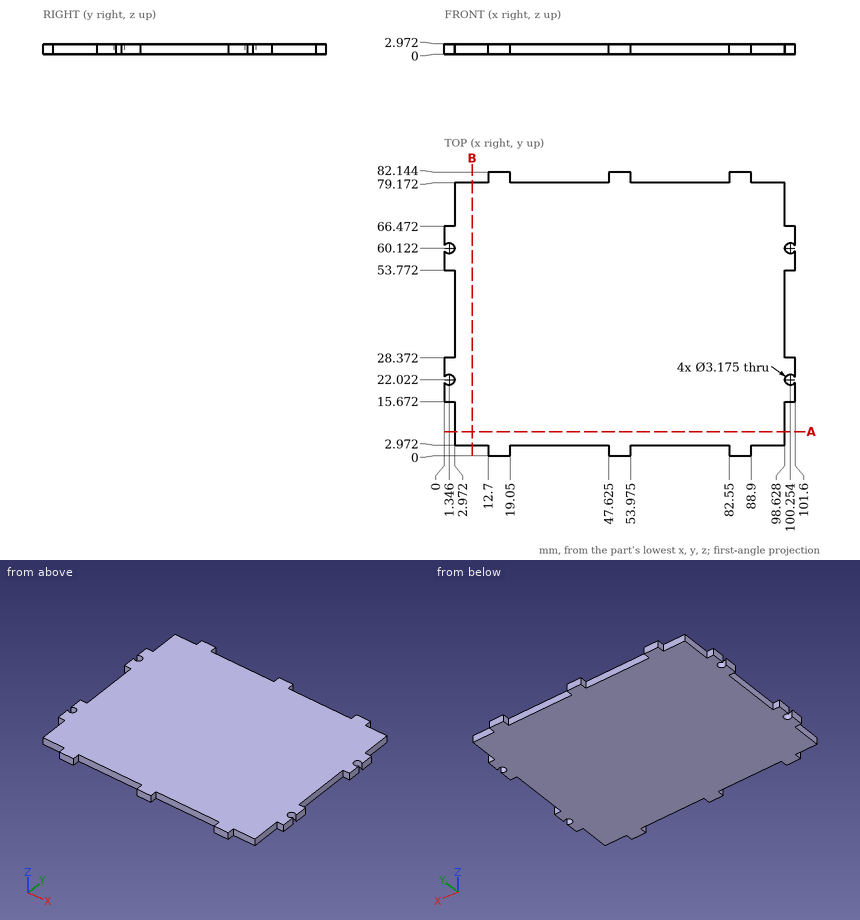
Print and shaded views of the part. All mm, measured from the part's lowest x, y and z. Coordinates: 2 decimals unless noted, no trailing zeros. Write each loop counter-clockwise with the first axis right and the second up, starting at its lowest first coordinate (ties: lowest second). Pieces come first, ordered by that corner, then holes.
(1) Cut at A-A, the plane y = 7. List the corners of the cut face in (x, z).
(2) Drill centre lines: probe 1 along X at (y, z) = (69, 1.9); probe 2 along Y at (x, z) = (60.5, 1.1). Where is each one in solid material? Low to high.
(3) Flat gauge pins, fed straight in: pin 1 (1.5 mm diameter, centred on y = 1.5, z = 2, fed in from -X); pin 2 (1.5 mm diameter, centred on x = 100, z = 1, fed in from -Y); pin 3 (2 mm diameter, centred on x = 80.5, y = 28.5, fed in from -Z); pin 4 (1.5 mm diameter, centred on y = 36.5, z = 2, fed in from -X). Where does each tip first touch, or does it go through?
(4) Cut at B-B, the plane x = 8. List the corners of the cut face in (y, z).
Geometry says:
1. outline: (2.97, 0) - (98.63, 0) - (98.63, 2.97) - (2.97, 2.97) - close
2. probe 1: x = 2.97 to 98.63
2. probe 2: y = 2.97 to 79.17
3. pin 1: stops at x = 12.7
3. pin 2: stops at y = 15.67
3. pin 3: stops at z = 0
3. pin 4: stops at x = 2.97
4. outline: (2.97, 0) - (79.17, 0) - (79.17, 2.97) - (2.97, 2.97) - close
